from build123d import *

# Parameters (mm, degrees)
F0_W     = 22
F0_H     = 70
F1_DEPTH = 3
F0_W_2   = 109
F0_H_2   = 25
F0_H_3   = 30
F0_W_3   = 10
F2_DEPTH = 20
F0_H_4   = 5
F3_DEPTH = 6
F4_R     = 4.99999
F5_R     = 5
F6_R     = 2


# Not quite as in the source:
# - a fillet or chamfer is up to 0.001 mm smaller than in the source, because OpenCascade refuses the exact size


with BuildPart() as f1:
    # F0 (on Top) → F1 (new body)
    with BuildSketch(Plane.XY):
        with Locations((-111.672727108, 5)):
            Rectangle(F0_W, F0_H)
    extrude(amount=F1_DEPTH)



with BuildPart() as f1b:
    # F0 (on Top) → F1, piece 2 (new body)
    with BuildSketch(Plane.XY):
        with Locations((39.327272892, 5)):
            Rectangle(F0_W, F0_H)
    extrude(amount=F1_DEPTH)


with BuildPart() as f1c:
    # F0 (on Top) → F1, piece 3 (new body)
    with BuildSketch(Plane.XY):
        with Locations((-36.172727108, 22.5)):
            Rectangle(F0_W_2, F0_H_2)
    extrude(amount=F1_DEPTH)


with BuildPart() as f1d:
    # F0 (on Top) → F1, piece 4 (new body)
    with BuildSketch(Plane.XY):
        with Locations((-36.172727108, -10)):
            Rectangle(F0_W_2, F0_H_3)
    extrude(amount=F1_DEPTH)


with BuildPart() as f1_1:
    add(f1.part)

    add(f1b.part)  # F2 merges F1b

    add(f1c.part)  # F2 merges F1c

    add(f1d.part)  # F2 merges F1d
    # F0 (on Top) → F2 (join)
    with BuildSketch(Plane.XY):
        with Locations((55.327272892, 5)):
            Rectangle(F0_W_3, F0_H)
        with Locations((-127.672727108, 5)):
            Rectangle(F0_W_3, F0_H)
        Polygon((-100.672727108, -30), (-90.672727108, -30), (-90.672727108, -25), (-90.672727108, 5), (-90.672727108, 10), (-90.672727108, 35), (-90.672727108, 40), (-100.672727108, 40), align=None)
        Polygon((18.327272892, -30), (28.327272892, -30), (28.327272892, 40), (18.327272892, 40), (18.327272892, 35), (18.327272892, 10), (18.327272892, 5), (18.327272892, -25), align=None)
    extrude(amount=F2_DEPTH)

    # F0 (on Top) → F3 (join)
    with BuildSketch(Plane.XY):
        with Locations((-36.172727108, 7.5)):
            Rectangle(F0_W_2, F0_H_4)
        with Locations((-36.172727108, -27.5)):
            Rectangle(F0_W_2, F0_H_4)
        with Locations((-36.172727108, 37.5)):
            Rectangle(F0_W_2, F0_H_4)
    extrude(amount=F3_DEPTH)

    # F4 (radius 5 in the source; OpenCascade refuses exactly that, so slightly less here)
    f4_edges = [f1_1.edges().sort_by_distance(p)[0] for p in [
        (50.327273, 5, 20),
        (28.327273, 5, 20),
        (-100.672727, 5, 20),
        (-122.672727, 5, 20),
        (-132.672727, 5, 20),
        (-90.672727, 5, 20),
        (18.327273, 5, 20),
        (60.327273, 5, 20),
    ]]
    fillet(f4_edges, radius=F4_R)

    # F5
    f5_edges = [f1_1.edges().sort_by_distance(p)[0] for p in [
        (-132.672727, 5, 0),
        (60.327273, 5, 0),
    ]]
    fillet(f5_edges, radius=F5_R)

    # F6
    f6_edges = [f1_1.edges().sort_by_distance(p)[0] for p in [
        (-36.172727, 5, 6),
        (-36.172727, 10, 6),
        (-36.172727, -30, 6),
        (-36.172727, 40, 6),
        (-36.172727, 35, 6),
        (-36.172727, -25, 6),
    ]]
    fillet(f6_edges, radius=F6_R)


solid = f1_1.part
Check sheet for the modelled part. Datum: model origin and axes. Units: mm. A direction names the side the tool comes from. Round coordinates to 2 decimals unless told otherwise and drop trailing zeros. Loops run counter-clockwise (first coordinate to the right, second up) from the corner with the lowest first, then second, coordinate; pieces in that order, holes last.
1. Set-up check for faces 4 (the flat face through (50.327, 5, 9)), 5 (the cylindrical face through (-131.169, 5.49, 1.426)), 6 (the flat face through (18.327, 5, 9)): record each of +Z, -Z, +X, -X, +Y, -Y from which the full face is reachable in a straight line by a thin tool's end or side.
2. Sectioned sample at D-D on z = 17. Record the boundary of the cut face in (x, y).
3. Sectioned sample at A-A on z = 8.5. Record the boundary of the cut face in (x, y), and give its area (3 significant figures).
4. Mould release check, pull along Y, two halves, no side actions. Record for faces 1 (the flat face through (-29, -30, 3)), 2 (the flat face through (-37, -10, 3)), 3 (the flat face through (-29, 40, 3)): released by +Y, released by -Y, zero draft, split by the parting line, or undercut.
5. Sectioned sample at C-C on x = -50.5. Record the boundary of the cut face in (y, z).
6. Gauge pin test, flat ends, axial feed: pin 1 Ø24 at (x, y) = (-39.5, -11) entering from +Z; pin 2 Ø0.8 at (x, y) = (-39.5, 7.5) entering from +Z; pin 3 Ø1 at (x, z) = (-89, 17.5) entering from +Y. Record the tip position at first contact, or that the pin passes through.
7. Scan lines: probe 1 along X at (y, z) = (33.5, 12.75); probe 2 along X at (y, z) = (36, 18.5); probe 3 along Z at (x, y) = (-118.5, -14). Record each from-to range of solid material in increasing order.
Recorded:
1. face 4: +Z, +Y, -Y
1. face 5: -Z, -X, +Y, -Y
1. face 6: +Z
2. outline: (-132.26, -30) - (-123.09, -30) - (-123.09, 40) - (-132.26, 40) - close; (-100.26, -30) - (-91.09, -30) - (-91.09, 40) - (-100.26, 40) - close; (18.74, -30) - (27.91, -30) - (27.91, 40) - (18.74, 40) - close; (50.74, -30) - (59.91, -30) - (59.91, 40) - (50.74, 40) - close
3. outline: (-132.67, -30) - (-122.67, -30) - (-122.67, 40) - (-132.67, 40) - close; (-100.67, -30) - (-90.67, -30) - (-90.67, 40) - (-100.67, 40) - close; (18.33, -30) - (28.33, -30) - (28.33, 40) - (18.33, 40) - close; (50.33, -30) - (60.33, -30) - (60.33, 40) - (50.33, 40) - close
3. area: 2,800 mm2
4. face 1: released by -Y
4. face 2: undercut
4. face 3: released by +Y
5. outline: (-30, 0) - (40, 0) - (40, 4) arc R2 ccw to (38, 6) - (37, 6) arc R2 ccw to (35, 4) - (35, 3) - (10, 3) - (10, 4) arc R2 ccw to (8, 6) - (7, 6) arc R2 ccw to (5, 4) - (5, 3) - (-25, 3) - (-25, 4) arc R2 ccw to (-27, 6) - (-28, 6) arc R2 ccw to (-30, 4) - close
6. pin 1: stops at z = 3
6. pin 2: stops at z = 6
6. pin 3: passes through
7. probe 1: x = -132.67 to -122.67, -100.67 to -90.67, 18.33 to 28.33, 50.33 to 60.33
7. probe 2: x = -131.24 to -124.1, -99.24 to -92.1, 19.76 to 26.9, 51.76 to 58.9
7. probe 3: z = 0 to 3
